```python
from build123d import *

# Parameters (mm, degrees)
SKETCH_1_R      = 1.5
EXTRUDE_1_DEPTH = 3
FILLET_1_R      = 3


with BuildPart() as part:
    # 草图1 → 凸台-拉伸1 (new body)
    with BuildSketch(Plane.XY):
        with BuildLine():
            Line((-85, -14), (0, -14))
            ThreePointArc((0, -14), (14, 0), (0, 14))
            Line((0, 14), (-85, 14))
            Line((-85, 14), (-85, -14))
        make_face()
        with Locations((-54.5, -11.5)):
            Circle(SKETCH_1_R, mode=Mode.SUBTRACT)
        with Locations((-77.5, -11.5)):
            Circle(SKETCH_1_R, mode=Mode.SUBTRACT)
        with Locations((-66, 0)):
            Circle(SKETCH_1_R, mode=Mode.SUBTRACT)
        with Locations((0, -8)):
            Circle(SKETCH_1_R, mode=Mode.SUBTRACT)
        with Locations((8, 0)):
            Circle(SKETCH_1_R, mode=Mode.SUBTRACT)
        with Locations((-77.5, 11.5)):
            Circle(SKETCH_1_R, mode=Mode.SUBTRACT)
        with Locations((-54.5, 11.5)):
            Circle(SKETCH_1_R, mode=Mode.SUBTRACT)
        with Locations((-8, 0)):
            Circle(SKETCH_1_R, mode=Mode.SUBTRACT)
        with Locations((0, 8)):
            Circle(SKETCH_1_R, mode=Mode.SUBTRACT)
    extrude(amount=EXTRUDE_1_DEPTH)

    # 圆角1
    fillet_1_edges = [part.edges().sort_by_distance(p)[0] for p in [
        (-85, 14, 1.5),
        (-85, -14, 1.5),
    ]]
    fillet(fillet_1_edges, radius=FILLET_1_R)


solid = part.part
```
Could you check a few things on this model? Use its own coordinates, in mm. Round coordinates to 2 decimals unless told otherwise and drop trailing zeros. Loops run counter-clockwise (first coordinate to the right, second up) from the corner with the lowest first, then second, coordinate; pieces in that order, holes last. Notation, with made-up numbers: (9.25, 39) -> (68.25, 39) arc R11 cw to (68.25, 57) -> close; hole circle Ø6 at (-0.75, -0.75). An arc over 180 degrees is marked (long way). One line per question, with ' | ' between items.
(1) If we section it at D-D on x = 8: List the corners of the cut face in (y, z) for me, and give its area (3 significant figures).
Model answer:
outline: (-11.49, 0) -> (-1.5, 0) -> (-1.5, 3) -> (-11.49, 3) -> close; (1.5, 0) -> (11.49, 0) -> (11.49, 3) -> (1.5, 3) -> close | area: 59.9 mm^2
(2) If we section it at A-A on x = -66: List the corners of the cut face in (y, z) for me.
Model answer:
outline: (-14, 0) -> (-1.5, 0) -> (-1.5, 3) -> (-14, 3) -> close; (1.5, 0) -> (14, 0) -> (14, 3) -> (1.5, 3) -> close
(3) If we section it at B-B on x = -77.5: List the corners of the cut face in (y, z) for me.
Model answer:
outline: (-14, 0) -> (-13, 0) -> (-13, 3) -> (-14, 3) -> close; (-10, 0) -> (10, 0) -> (10, 3) -> (-10, 3) -> close; (13, 0) -> (14, 0) -> (14, 3) -> (13, 3) -> close
(4) If I drill on probe 1 along Y at (x, z) = (-54.5, 1.5); probe 2 along Y at (x, z) = (0, 1.95); probe 3 along X at (y, z) = (-11, 1.75), over which ranges is the centre line in solid material (lowest first)?
Model answer:
probe 1: y = -14 to -13, -10 to 10, 13 to 14 | probe 2: y = -14 to -9.5, -6.5 to 6.5, 9.5 to 14 | probe 3: x = -85 to -78.91, -76.09 to -55.91, -53.09 to 8.66
(5) If we section it at C-C on z = 2.35: Count the separate pieces of the cut face and the enclosed holes in it, and give its area (3 significant figures).
Model answer:
separate pieces: 1 | enclosed holes: 9 | area: 2,620 mm^2
(6) Thinking about a two-plate mould opening in X: for faces 1 (the face through (-84.14, 13.1, 1.52)), 2 (the face through (-53.07, 11.95, 1.48)), 3 (the face through (-0.325, -9.464, 1.479)), 4 (the face through (-40, 14, 1)), which applies, released by +X, released by -X, zero draft, split by the parting line, or undercut?
Model answer:
face 1: released by -X | face 2: undercut | face 3: undercut | face 4: zero draft
